Part print with two shaded views. Sizes in mm from the minimum x, y, z corner. A direction names the side the tool comes from. Coordinates: 2 decimals unless noted, no trailing zeros. Loops run counter-clockwise (first coordinate to the right, second up) from the corner with the lowest first, then second, coordinate; pieces in that order, holes last. Notation, with made-up numbers: (65, -19) -> (73, -19) arc R17 ccw to (73, -7) -> close; hole circle Ø8 at (19.25, -25.75). An arc over 180 degrees is marked (long way). Return JSON: item names as keys, results as strings. Group by question number.
(1) Saw through at D-D on y = 28.5. Write the cut outline in (x, z), then the cut area to 3 significant figures.
(2) Probe L1, parallel to Y at x = 10, z = 3.7; L2, parallel to Y at x = 10.25, z = 1.5; L3, parallel to Y at x = 13.25, z = 7.75. List the from-to ranges inside material, lowest first.
(3) Saw through at B-B on x = 15.25. Write the cut outline in (y, z).
(4) Saw through at C-C on y = 54. Write the cut outline in (x, z).
(5) Mould opens along Y. For the marked faces 1, 2 and 3 say: pulls with the +Y half, pulls with the -Y half, needs draft (parallel to the pull), parting line crosses it, or undercut.
(6) Flat gauge pins, fed straight in: pin 1 Ø1 at (x, y) = (6.5, 53.5) entering from -Z; pin 2 Ø3 at (x, y) = (8.5, 43.5) entering from +Z; pin 3 Ø1.6 at (x, y) = (11, 56) entering from -Z; pin 4 Ø2 at (x, y) = (10, 5) entering from +Z. Where does each tip first touch, or does it go through?
(7) Saw through at A-A on z = 5. Write the cut outline in (x, y).
(8) Tool access for the marked faces 4 and 5: list every direction of +Z, -Z, +X, -X, +Y, -Y with a clear straight run to the whole face (end or side of a thin tool).
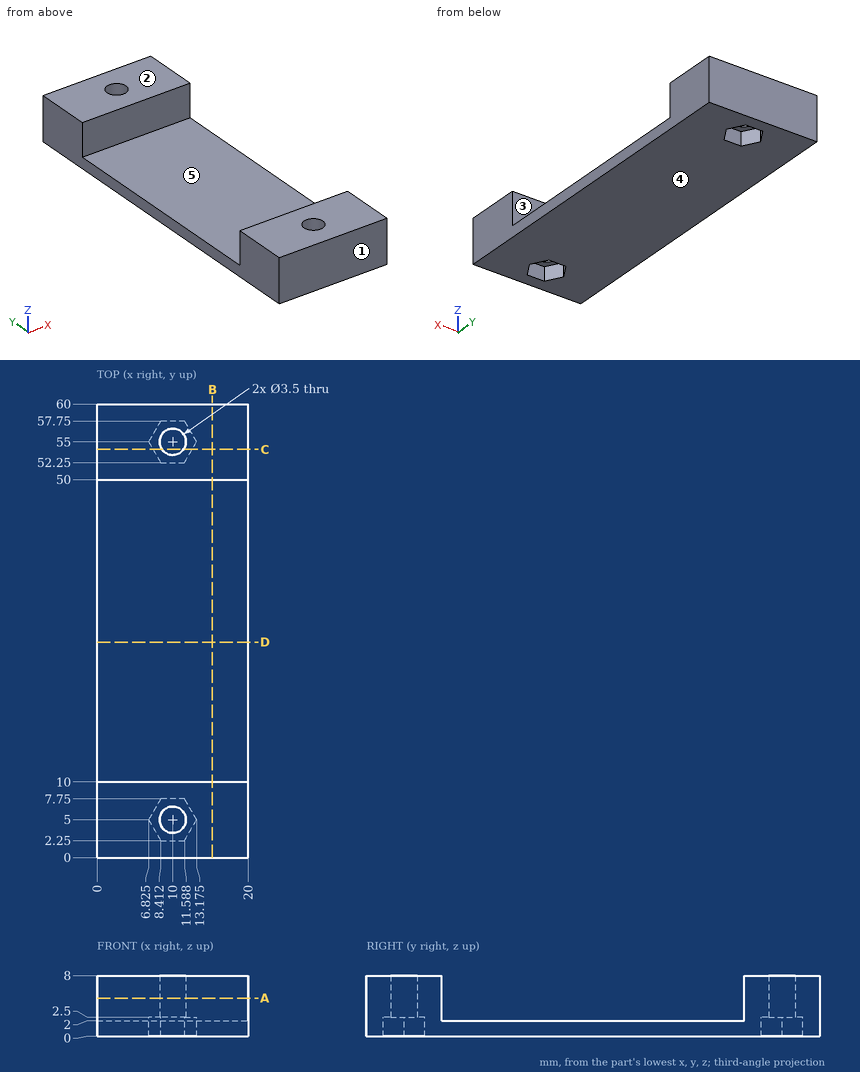
Geometry results:
{
 "1": {"outline": "(0, 0) -> (20, 0) -> (20, 2) -> (0, 2) -> close", "area": "40.0 mm²"},
 "2": {"L1": "0 to 3.25, 6.75 to 10, 50 to 53.25, 56.75 to 60", "L2": "0 to 2.25, 7.75 to 52.25, 57.75 to 60", "L3": "0 to 10, 50 to 60"},
 "3": {"outline": "(0, 0) -> (60, 0) -> (60, 8) -> (50, 8) -> (50, 2) -> (10, 2) -> (10, 8) -> (0, 8) -> close"},
 "4": {"outline": "(0, 0) -> (7.4, 0) -> (7.4, 2.5) -> (8.56, 2.5) -> (8.56, 8) -> (0, 8) -> close; (11.44, 2.5) -> (12.6, 2.5) -> (12.6, 0) -> (20, 0) -> (20, 8) -> (11.44, 8) -> close"},
 "5": {"face 1": "pulls with the -Y half", "face 2": "needs draft", "face 3": "undercut"},
 "6": {"pin 1": "z = 0", "pin 2": "z = 2", "pin 3": "z = 2.5", "pin 4": "through"},
 "7": {"outline": "(0, 0) -> (20, 0) -> (20, 10) -> (0, 10) -> close; (0, 50) -> (20, 50) -> (20, 60) -> (0, 60) -> close; hole circle Ø3.5 at (10, 5); hole circle Ø3.5 at (10, 55)"},
 "8": {"face 4": "-Z, +X, -X, +Y, -Y", "face 5": "+Z, +X, -X"}
}
